```python
from build123d import *

# Parameters (mm, degrees)
SKETCH1_W           = 16.0208
SKETCH1_H           = 7.8
SKETCH1_W_2         = 14.0208
SKETCH1_H_2         = 5.8
BOSS_EXTRUDE1_DEPTH = 0.9
BOSS_EXTRUDE2_START = -0.9
SKETCH1_4_W         = 14.0208
SKETCH1_4_H         = 5.8
BOSS_EXTRUDE2_DEPTH = 1.1


with BuildPart() as part:
    # Sketch1 → Boss-Extrude1 (new body)
    # profile 1 of 2: a face of its own
    with BuildSketch(Plane.XY):
        with Locations((-113.3983, -100.1518)):
            Rectangle(SKETCH1_W, SKETCH1_H)
        with Locations((-113.3983, -100.1518)):
            Rectangle(SKETCH1_W_2, SKETCH1_H_2, mode=Mode.SUBTRACT)
    # profile 2 of 2: a face of its own
    with BuildSketch(Plane.XY):
        with Locations((-113.3983, -100.1518)):
            Rectangle(SKETCH1_W_2, SKETCH1_H_2)
    extrude(amount=-BOSS_EXTRUDE1_DEPTH)

    # Sketch1<4> → Boss-Extrude2 (add)
    with BuildSketch(Plane.XY.offset(BOSS_EXTRUDE2_START)):
        with Locations((-113.3983, -100.1518)):
            Rectangle(SKETCH1_4_W, SKETCH1_4_H)
    extrude(amount=-BOSS_EXTRUDE2_DEPTH)


solid = part.part
```
CAD build for the part. Positions are in the model's coordinates, mm. A direction names the side the tool comes from. Coordinates: 2 decimals unless noted, no trailing zeros. Order: outer loops, then holes, each group sorted by start corner. A loop starts at its lowest first (then second) coordinate and runs counter-clockwise, first axis right, second up.
(1) Drill centre lines: L1, parallel to Y at x = -110, z = -1.5; L2, parallel to X at y = -101.75, z = -1.65; L3, parallel to Z at x = -116.75, y = -96.75. Where is each one in solid material? Low to high.
Solution:
L1: y = -103.05 to -97.25
L2: x = -120.41 to -106.39
L3: z = -0.9 to 0
(2) Mould opens along Y. For faces 3 (the face through (-113.5, -103.052, -1.4)), 4 (the face through (-113.5, -97.252, -1.4)), 5 (the face through (-106.388, -100.2, -1.4)) say: released by +Y, released by -Y, zero draft, split by the parting line, or undercut.
Solution:
face 3: released by -Y
face 4: released by +Y
face 5: zero draft
(3) Pin check, flat tip, straight feed: pin 1 Ø0.6 at (y, z) = (-99, -1.5) entering from +X. Stop position of the tip, or through.
Solution:
pin 1: stops at x = -106.39
(4) Saw through at A-A, the plane x = -114. Write the cut outline in (y, z).
Solution:
outline: (-104.05, -0.9) - (-103.05, -0.9) - (-103.05, -2) - (-97.25, -2) - (-97.25, -0.9) - (-96.25, -0.9) - (-96.25, 0) - (-104.05, 0) - close
(5) Which spindle directions (+Z, -Z, +X, -X, +Y, -Y) get a long thin tool onto all of the face, cutting with end or side? Do faces 1 (the face through (-120.409, -100.2, -1.4)), 2 (the face through (-114, -100, 0)). Say none if no direction does.
Solution:
face 1: -Z, -X, +Y, -Y
face 2: +Z, +X, -X, +Y, -Y
(6) Saw through at C-C, the plane z = -1.5. Write the cut outline in (x, y), and give its area (3 significant figures).
Solution:
outline: (-120.41, -103.05) - (-106.39, -103.05) - (-106.39, -97.25) - (-120.41, -97.25) - close
area: 81.3 mm2
(7) Saw through at B-B, the plane y = -101.5. Write the cut outline in (x, z).
Solution:
outline: (-121.41, -0.9) - (-120.41, -0.9) - (-120.41, -2) - (-106.39, -2) - (-106.39, -0.9) - (-105.39, -0.9) - (-105.39, 0) - (-121.41, 0) - close
(8) Saw through at D-D, the plane y = -96.5. Write the cut outline in (x, z), and give its area (3 significant figures).
Solution:
outline: (-121.41, -0.9) - (-105.39, -0.9) - (-105.39, 0) - (-121.41, 0) - close
area: 14.4 mm2
